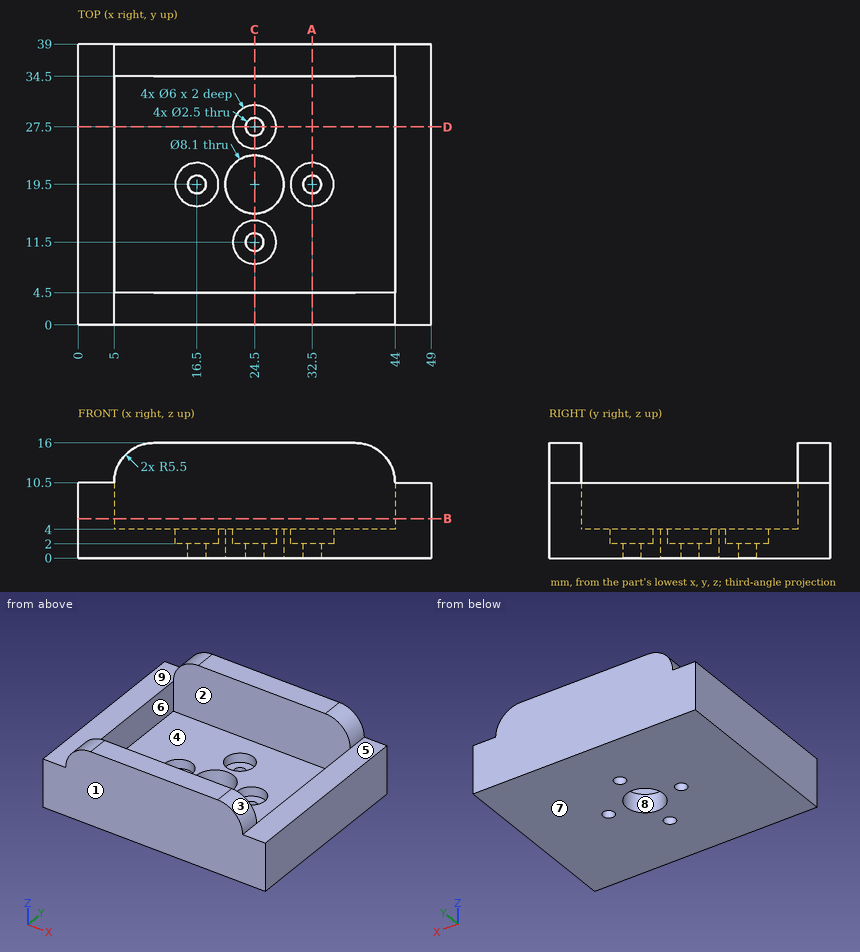
Here's the drawing with two shaded views (mm, measured from the low corner). I have some questions. A direction names the side the tool comes from. Coordinates: 2 decimals unless noted, no trailing zeros. Loops run counter-clockwise (first coordinate to the right, second up) from the corner with the lowest first, then second, coordinate; pieces in that order, holes last. Notation, with made-up numbers: M -28.5,80.5 L 9.5,80.5 A23 ccw 9.5,112.5 Z; hole C 84,16 d1. An arc over 180 degrees is marked long. Put each result on its own line as item: value. Start each with the question number.
(1) I need wall thicknesses on probe 1 along X at (y, z) = (19.5, 0.75); probe 2 along Y at (x, z) = (24.5, 2.55); probe 3 along X at (y, z) = (15.5, 7.25). Which ranges of each line are inside material? Lowest first, please.
(2) Which directions (+Z, -Z, +X, -X, +Y, -Y) give clear straight access to the entire face, cutting with the end or side of a thin tool? Please do the marked faces 5, 6, 7, 8 and 9.
(3) We'd pull the mould along Y, two halves only. Please class the marked faces 1, 2, 3 and 4: +Y half, -Y half, draft (parallel to the pull), parting line (faces both ways), or undercut.
(4) Will these pins go through, and if not, where does the flat tip stop? pin 1 Ø1.5 at (x, y) = (45.5, 28.5) entering from +Z; pin 2 Ø2 at (x, y) = (16.5, 19.5) entering from +Z (3 decimals); pin 3 Ø4 at (x, y) = (32.5, 19.5) entering from +Z; pin 4 Ø8 at (x, y) = (16.5, 19.5) entering from +Z.
(5) Imagine slicing it at A-A on x = 32.5. List the corners of the cut face in (y, z) for me.
(6) Imagine slicing it at B-B on z = 5.5. List the corners of the cut face in (x, y) for me, and give its area (3 significant figures).
(7) Imagine slicing it at D-D on y = 27.5. List the corners of the cut face in (x, z) for me, and give its area (3 significant figures).
(8) Imagine slicing it at C-C on x = 24.5. List the corners of the cut face in (y, z) for me.
Worked answers:
1. probe 1: x = 0 to 15.25, 17.75 to 20.45, 28.55 to 31.25, 33.75 to 49
1. probe 2: y = 0 to 8.5, 14.5 to 15.45, 23.55 to 24.5, 30.5 to 39
1. probe 3: x = 0 to 5, 44 to 49
2. face 5: +Z, +X, +Y, -Y
2. face 6: +Z
2. face 7: -Z, +X, -X, +Y, -Y
2. face 8: +Z, -Z
2. face 9: +Z, -X, +Y, -Y
3. face 1: -Y half
3. face 2: undercut
3. face 3: draft
3. face 4: undercut
4. pin 1: stops at z = 10.5
4. pin 2: passes through
4. pin 3: stops at z = 2
4. pin 4: stops at z = 4
5. outline: M 0,0 L 18.25,0 L 18.25,2 L 16.5,2 L 16.5,4 L 4.5,4 L 4.5,16 L 0,16 Z; M 20.75,0 L 39,0 L 39,16 L 34.5,16 L 34.5,4 L 22.5,4 L 22.5,2 L 20.75,2 Z
6. outline: M 0,0 L 49,0 L 49,39 L 0,39 Z; hole M 5,4.5 L 44,4.5 L 44,34.5 L 5,34.5 Z
6. area: 741 mm2
7. outline: M 0,0 L 23.25,0 L 23.25,2 L 21.5,2 L 21.5,4 L 5,4 L 5,10.5 L 0,10.5 Z; M 25.75,0 L 49,0 L 49,10.5 L 44,10.5 L 44,4 L 27.5,4 L 27.5,2 L 25.75,2 Z
7. area: 244 mm2
8. outline: M 0,0 L 10.25,0 L 10.25,2 L 8.5,2 L 8.5,4 L 4.5,4 L 4.5,16 L 0,16 Z; M 12.75,0 L 15.45,0 L 15.45,4 L 14.5,4 L 14.5,2 L 12.75,2 Z; M 23.55,0 L 26.25,0 L 26.25,2 L 24.5,2 L 24.5,4 L 23.55,4 Z; M 28.75,0 L 39,0 L 39,16 L 34.5,16 L 34.5,4 L 30.5,4 L 30.5,2 L 28.75,2 Z
